Source: CAD feature listing. Evaluate the final solid. Frame: model axes, mm. A direction names the side the tool comes from. Round coordinates to 2 decimals unless told otherwise and drop trailing zeros. Loops run counter-clockwise (first coordinate to the right, second up) from the corner with the lowest first, then second, coordinate; pieces in that order, holes last. Notation, with made-up numbers: M 70.25,-25.5 L 121.25,-25.5 A9 cw 121.25,-21.5 Z; hole C 1.5,37 d2. An arc over 180 degrees is marked long. Answer as a JSON object with one key per item and string values.
from build123d import *

# Parameters (mm, degrees)
BOX002_W       = 13
BOX002_H       = 25
BOX002_DEPTH   = 3
BOX001_W       = 13
BOX001_H       = 25
BOX001_DEPTH   = 3
CYLINDER_R     = 4
CYLINDER_DEPTH = 3
BOX_W          = 100
BOX_H          = 100
BOX_DEPTH      = 3


with BuildPart() as cube002:
    # Box002 → Box002 (new body)
    with BuildSketch(Plane(origin=(-46, -12, 0), x_dir=(1, 0, 0), z_dir=(0, 0, 1))):
        with Locations((6.5, 12.5)):
            Rectangle(BOX002_W, BOX002_H)
    extrude(amount=BOX002_DEPTH)


with BuildPart() as cube001:
    # Box001 → Box001 (new body)
    with BuildSketch(Plane(origin=(34, -12, 0), x_dir=(1, 0, 0), z_dir=(0, 0, 1))):
        with Locations((6.5, 12.5)):
            Rectangle(BOX001_W, BOX001_H)
    extrude(amount=BOX001_DEPTH)


with BuildPart() as cylinder:
    # Cylinder → Cylinder (new body)
    with BuildSketch(Plane.XY):
        Circle(CYLINDER_R)
    extrude(amount=CYLINDER_DEPTH)


with BuildPart() as cut002:
    # Box → Box (new body)
    with BuildSketch(Plane(origin=(-50, -50, 0), x_dir=(1, 0, 0), z_dir=(0, 0, 1))):
        with Locations((50, 50)):
            Rectangle(BOX_W, BOX_H)
    extrude(amount=BOX_DEPTH)

    # Cut: cut Cylinder
    add(cylinder.part, mode=Mode.SUBTRACT)

    # Cut001: cut Cube001
    add(cube001.part, mode=Mode.SUBTRACT)

    # Cut002: cut Cube002
    add(cube002.part, mode=Mode.SUBTRACT)


solid = cut002.part
Item 1: Section D-D on x = 0. Return the cut outline in (y, z), then the cut area to 3 significant figures.
Answer sheet:
{"outline": "M -50,0 L -4,0 L -4,3 L -50,3 Z; M 4,0 L 50,0 L 50,3 L 4,3 Z", "area": "276 mm²"}
Item 2: Pull-direction query (Y, two-part tool) for faces 1 (the flat face through (-40, 13, 1)), 2 (the flat face through (-1, 50, 1)), 3 (the flat face through (-50, -1, 1)); classes: pulls with the +Y half, pulls with the -Y half, needs draft (parallel to the pull), parting line crosses it, or undercut.
Answer sheet:
{"face 1": "undercut", "face 2": "pulls with the +Y half", "face 3": "needs draft"}
Item 3: Section A-A on x = -35. Return the cut outline in (y, z), then the cut area to 3 significant figures.
Answer sheet:
{"outline": "M -50,0 L -12,0 L -12,3 L -50,3 Z; M 13,0 L 50,0 L 50,3 L 13,3 Z", "area": "225 mm²"}
Item 4: Section B-B on y = 0. Return the cut outline in (x, z), then the cut area to 3 significant figures.
Answer sheet:
{"outline": "M -50,0 L -46,0 L -46,3 L -50,3 Z; M -33,0 L -4,0 L -4,3 L -33,3 Z; M 4,0 L 34,0 L 34,3 L 4,3 Z; M 47,0 L 50,0 L 50,3 L 47,3 Z", "area": "198 mm²"}
Item 5: Line query: probe 1 along X at (y, z) = (11, 0.35); probe 2 along Y at (x, z) = (0, 2.25); probe 3 along Y at (x, z) = (-34, 1.1). Output: solid intervals per line, ascending. Write a range as from..to.
Answer sheet:
{"probe 1": "x = -50..-46, -33..34, 47..50", "probe 2": "y = -50..-4, 4..50", "probe 3": "y = -50..-12, 13..50"}
Item 6: Access query for faces 4 (the flat face through (40, 13, 1)), 5 (the flat face through (10, 1, 0)). Directions: +Z, -Z, +X, -X, +Y, -Y. A direction counts if a zero-diameter tool reaches every point of the face in a straight line with its end or side. Return the directions, or none.
Answer sheet:
{"face 4": "+Z, -Z", "face 5": "-Z, +X, -X, +Y, -Y"}
Item 7: Section C-C on z = 2. Return the cut outline in (x, y), then the cut area to 3 significant figures.
Answer sheet:
{"outline": "M -50,-50 L 50,-50 L 50,50 L -50,50 Z; hole M -46,-12 L -33,-12 L -33,13 L -46,13 Z; hole C 0,0 d8; hole M 34,-12 L 47,-12 L 47,13 L 34,13 Z", "area": "9,300 mm²"}
Item 8: Contact query for a flat-ended pin moving along its axis: pin 1 Ø1.5 at (x, y) = (36, -5.5) entering from -Z. Output: stop coordinate, or through.
Answer sheet:
{"pin 1": "passes through"}
